```python
from build123d import *

# Parameters (mm, degrees)
SKETCH1_R           = 25.000012525
SKETCH1_R_2         = 5
BOSS_EXTRUDE1_DEPTH = 10
SKETCH3_R           = 2.5
CUT_EXTRUDE1_DEPTH  = 16
SKETCH4_R           = 2.5
CUT_EXTRUDE2_DEPTH  = 16
FILLET1_R           = 5
FILLET2_R           = 5


with BuildPart() as part:
    # Sketch1 → Boss-Extrude1 (new body)
    with BuildSketch(Plane(origin=(0, 0, 0), x_dir=(1, 0, 0), z_dir=(0, 1, 0))):
        with BuildLine():
            Line((-70, -30.387602841), (-39.706341981, -30.387602841))
            ThreePointArc((-39.706341981, -30.387602841), (0, 50), (39.706341981, -30.387602841))
            Line((39.706341981, -30.387602841), (70, -30.387602841))
            Line((70, -30.387602841), (70, -45.387602841))
            Line((70, -45.387602841), (48, -45.387602841))
            Line((48, -45.387602841), (48, -40.387602841))
            Line((48, -40.387602841), (-48, -40.387602841))
            Line((-48, -40.387602841), (-48, -45.387602841))
            Line((-48, -45.387602841), (-70, -45.387602841))
            Line((-70, -45.387602841), (-70, -30.387602841))
        make_face()
        Circle(SKETCH1_R, mode=Mode.SUBTRACT)
        with Locations((30.781735211, 19.572623378)):
            Circle(SKETCH1_R_2, mode=Mode.SUBTRACT)
        with Locations((-30.781735211, 19.572623378)):
            Circle(SKETCH1_R_2, mode=Mode.SUBTRACT)
    extrude(amount=BOSS_EXTRUDE1_DEPTH)

    # Sketch3 → Cut-Extrude1 (cut, through all)
    with BuildSketch(Plane(origin=(0, 0, 30.387602841), x_dir=(-1, 0, 0), z_dir=(0, 0, -1))):
        with Locations((-63, 5)):
            Circle(SKETCH3_R)
    extrude(amount=-CUT_EXTRUDE1_DEPTH, mode=Mode.SUBTRACT)

    # Sketch4 → Cut-Extrude2 (cut, through all)
    with BuildSketch(Plane(origin=(0, 0, 30.387602841), x_dir=(-1, 0, 0), z_dir=(0, 0, -1))):
        with Locations((63, 5)):
            Circle(SKETCH4_R)
    extrude(amount=-CUT_EXTRUDE2_DEPTH, mode=Mode.SUBTRACT)

    # Fillet1
    fillet1_edges = [part.edges().sort_by_distance(p)[0] for p in [
        (39.706341981, 5, 30.387602841),
    ]]
    fillet(fillet1_edges, radius=FILLET1_R)

    # Fillet2
    fillet2_edges = [part.edges().sort_by_distance(p)[0] for p in [
        (-39.706341981, 5, 30.387602841),
    ]]
    fillet(fillet2_edges, radius=FILLET2_R)


solid = part.part
```
Work out the finished part from the listing and answer in its coordinate system (mm). A direction names the side the tool comes from. Give positions to 0.01 mm unless a question says otherwise; leave off trailing zeros. Loops run counter-clockwise (first coordinate to the right, second up) from the corner with the lowest first, then second, coordinate; pieces in that order, holes last. Notation, with made-up numbers: (45.25, 7) -> (73.25, 7) arc R21 ccw to (73.25, 22) -> close; hole circle Ø6 at (44.25, -30.5). An arc over 180 degrees is marked (long way). Put each result on its own line as item: value. Start each with the question number.
Item 1: The mould has two halves that part along Z. Classify faces 1 (the face through (-59, 5, 45.388)), 2 (the face through (-48, 5, 43)), 3 (the face through (-31.43, 4.93, -24.53)), 4 (the face through (-20, 5, 15)): released by +Z, released by -Z, zero draft, split by the parting line, or undercut.
Item 2: Find the intervals of material crossed by L1, parallel to Z at x = 0, y = 6.75; L2, parallel to X at y = 3, z = 35; L3, parallel to X at y = 9, z = 41.5, in increasing order. Write a range as [from, to].
Item 3: The part is cut by section B-B (x = -63). Give the vertices of the cut face in (y, z), then the cut area to 3 significant figures.
Item 4: Each of these flat-tipped pins is pushed along its axis until it touches: P1, Ø1.5, axis at x = -38.5, y = 4.5, coming from the -Z side; P2, Ø13, axis at x = -30.78, z = -19.57, coming from the -Y side; P3, Ø3, axis at x = -60, y = 4, coming from the -Z side; P4, Ø5, axis at x = 11.5, y = 7, coming from the +Z side. Where does it stop, or does it pass through?
Item 5: The part is cut by section D-D (x = 52). Give the vertices of the cut face in (y, z), then the cut area to 3 significant figures.
Item 6: The part is cut by section A-A (z = 0). Give the vertices of the cut face in (x, y).
Item 7: Which of the six approach directions +Z, -Z, +X, -X, +Y, -Y give full straight-line access (tool end or side, diameter ignored) to faces 5 (the face through (70, 5, 38)), 6 (the face through (48, 5, 43))?
Item 8: The part is cut by section C-C (y = 5). Give the vertices of the cut face in (x, z), then the cut area to 3 significant figures.
Answers below:
1. face 1: released by +Z
1. face 2: zero draft
1. face 3: undercut
1. face 4: undercut
2. L1: [-50, -25], [25, 40.39]
2. L2: [-70, -64.5], [-61.5, 61.5], [64.5, 70]
2. L3: [-70, -48], [48, 70]
3. outline: (0, 30.39) -> (2.5, 30.39) -> (2.5, 45.39) -> (0, 45.39) -> close; (7.5, 30.39) -> (10, 30.39) -> (10, 45.39) -> (7.5, 45.39) -> close
3. area: 75.0 mm2
4. P1: z = -32.79
4. P2: y = 0
4. P3: z = 30.39
4. P4: z = 40.39
5. outline: (0, 30.39) -> (10, 30.39) -> (10, 45.39) -> (0, 45.39) -> close
5. area: 150 mm2
6. outline: (-50, 0) -> (-25, 0) -> (-25, 10) -> (-50, 10) -> close; (25, 0) -> (50, 0) -> (50, 10) -> (25, 10) -> close
7. face 5: +Z, -Z, +X, +Y, -Y
7. face 6: +Z, +Y, -Y
8. outline: (-70, 30.39) -> (-65.5, 30.39) -> (-65.5, 45.39) -> (-70, 45.39) -> close; (-60.5, 30.39) -> (-48.79, 30.39) arc R5 cw to (-44.35, 23.08) arc R50 ccw (long way) to (44.35, 23.08) arc R5 cw to (48.79, 30.39) -> (60.5, 30.39) -> (60.5, 45.39) -> (48, 45.39) -> (48, 40.39) -> (-48, 40.39) -> (-48, 45.39) -> (-60.5, 45.39) -> close; (65.5, 30.39) -> (70, 30.39) -> (70, 45.39) -> (65.5, 45.39) -> close; hole circle Ø10 at (-30.78, -19.57); hole circle Ø50 at (0, 0); hole circle Ø10 at (30.78, -19.57)
8. area: 6,150 mm2
